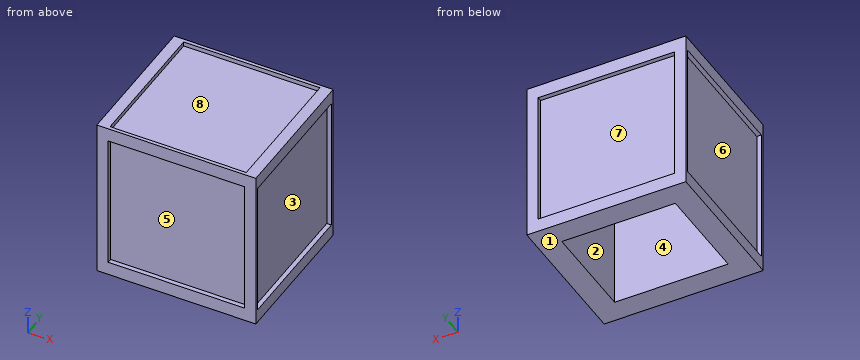
Autodesk Inventor part; units mm, degrees
ref_plane "YZ Plane" through (0, 0, 0) normal (1, 0, 0) x (0, 1, 0)
ref_plane "XZ Plane" through (0, 0, 0) normal (0, 1, 0) x (-1, 0, 0)
ref_plane "XY Plane" through (0, 0, 0) normal (0, 0, 1) x (1, 0, 0)
sketch "Sketch3" plane through (0, 0, 0) normal (0, 0, 1) x (1, 0, 0)
  line L0 (0, 0) -> (-50, 0)
  line L1 (-50, 0) -> (-50, 43)
  line L2 (-50, 43) -> (0, 43)
  line L3 (0, 43) -> (0, 0)
  line L4 (10, -10) -> (-60, -10)
  line L5 (-60, -10) -> (-60, 53)
  line L6 (-60, 53) -> (10, 53)
  line L7 (10, 53) -> (10, -10)
  dimension "d26" = 43
  dimension "d27" = 50
  dimension "d28" = 70
  dimension "d29" = 63
extrude "Extrusion3" add sketch "Sketch3" along normal blind 60
sketch "Sketch4" plane through (0, 0, 60) normal (0, 0, 1) x (1, 0, 0)
  line L0 (10, -10) -> (-60, -10)
  line L1 (-60, -10) -> (-60, 53)
  line L2 (-60, 53) -> (10, 53)
  line L3 (10, 53) -> (10, -10)
  point P0 (0, 0)
extrude "Extrusion4" add sketch "Sketch4" along normal blind 12
sketch "Sketch5" plane through (-60, 53, 0) normal (0, 1, 0) x (1, 0, 0)
  line L0 (0, 0) -> (70, 0)
  line L1 (70, 0) -> (70, -72)
  line L2 (0, 0) -> (70, 0)
  line L3 (70, 0) -> (70, -72)
  line L4 (70, -72) -> (0, -72)
  line L5 (0, -72) -> (0, 0)
  line L6 (65, -6) -> (5, -6)
  line L7 (5, -6) -> (5, -66)
  line L8 (5, -66) -> (65, -66)
  line L9 (65, -66) -> (65, -6)
  line L10 (60, -11) -> (10, -11)
  line L11 (10, -11) -> (10, -61)
  line L12 (10, -61) -> (60, -61)
  line L13 (60, -61) -> (60, -11)
  point P0 (60, 0)
  dimension "d34" = 60
  dimension "d35" = 60
  dimension "d36" = 50
  dimension "d37" = 50
extrude "Extrusion5" cut sketch "Sketch5" against normal blind 2 contours L9 L8 L7 L6 | L13 L12 L11 L10
sketch "Sketch6" plane through (10, -10, 0) normal (1, 0, 0) x (0, 0, -1)
  line L0 (-6, 1.5) -> (-66, 1.5)
  line L1 (-66, 1.5) -> (-66, 61.5)
  line L2 (-66, 61.5) -> (-6, 61.5)
  line L3 (-6, 61.5) -> (-6, 1.5)
  line L4 (-11, 6.5) -> (-61, 6.5)
  line L5 (-61, 6.5) -> (-61, 56.5)
  line L6 (-61, 56.5) -> (-11, 56.5)
  line L7 (-11, 56.5) -> (-11, 6.5)
  point P0 (0, 10)
  dimension "d40" = 60
  dimension "d41" = 60
  dimension "d42" = 50
  dimension "d43" = 50
extrude "Extrusion6" cut sketch "Sketch6" against normal blind 2 contours L0 L1 L2 L3 | L4 L5 L6 L7
sketch "Sketch7" plane through (-60, -10, 0) normal (0, -1, 0) x (1, 0, 0)
  line L0 (5, 6) -> (65, 6)
  line L1 (65, 6) -> (65, 66)
  line L2 (65, 66) -> (5, 66)
  line L3 (5, 66) -> (5, 6)
  line L4 (10, 11) -> (60, 11)
  line L5 (60, 11) -> (60, 61)
  line L6 (60, 61) -> (10, 61)
  line L7 (10, 61) -> (10, 11)
  point P0 (60, 0)
  dimension "d46" = 60
  dimension "d47" = 60
  dimension "d48" = 50
  dimension "d49" = 50
extrude "Extrusion7" cut sketch "Sketch7" against normal blind 2 contours L3 L2 L1 L0 | L7 L6 L5 L4
sketch "Sketch8" plane through (-60, -10, 0) normal (-1, 0, 0) x (0, 0, 1)
  line L0 (6, 1.5) -> (66, 1.5)
  line L1 (66, 1.5) -> (66, 61.5)
  line L2 (66, 61.5) -> (6, 61.5)
  line L3 (6, 61.5) -> (6, 1.5)
  line L4 (11, 6.5) -> (61, 6.5)
  line L5 (61, 6.5) -> (61, 56.5)
  line L6 (61, 56.5) -> (11, 56.5)
  line L7 (11, 56.5) -> (11, 6.5)
  point P0 (0, 10)
  dimension "d52" = 60
  dimension "d53" = 60
  dimension "d54" = 50
  dimension "d55" = 50
extrude "Extrusion8" cut sketch "Sketch8" against normal blind 2 contours L3 L2 L1 L0 | L7 L6 L5 L4
sketch "Sketch9" plane through (0, 0, 72) normal (0, 0, 1) x (1, 0, 0)
  line L0 (5, -8.5) -> (-55, -8.5)
  line L1 (-55, -8.5) -> (-55, 51.5)
  line L2 (-55, 51.5) -> (5, 51.5)
  line L3 (5, 51.5) -> (5, -8.5)
  line L4 (0, 46.5) -> (-50, 46.5)
  line L5 (-50, 46.5) -> (-50, -3.5)
  line L6 (-50, -3.5) -> (0, -3.5)
  line L7 (0, -3.5) -> (0, 46.5)
  point P0 (0, 0)
  dimension "d58" = 60
  dimension "d59" = 60
  dimension "d60" = 50
  dimension "d61" = 50
extrude "Extrusion9" cut sketch "Sketch9" against normal blind 2 contours L0 L1 L2 L3 | L7 L6 L5 L4
properties part number "End-Effector"
Work out the finished part from the listing and answer in its coordinate system (mm). Face numbers are marked on the shaded views. A direction names the side the tool comes from. Round coordinates to 2 decimals unless told otherwise and drop trailing zeros. Loops run counter-clockwise (first coordinate to the right, second up) from the corner with the lowest first, then second, coordinate; pieces in that order, holes last. Notation, with made-up numbers: (1, 52.5) - (58, 52.5) arc R13 cw to (58, 76.5) - close; hole circle Ø5 at (-20, -6.5). An arc over 180 degrees is marked (long way). One line per item, written item: value.
Q1. Straight lines are drawn through the part: probe 1 along Y at (x, z) = (-26, 22); probe 2 along X at (y, z) = (40, 53); probe 3 along X at (y, z) = (-2.5, 50). For each, find the intervals that lie inside material, in ascending order.
Check values:
probe 1: -8 to 0, 43 to 51
probe 2: -58 to -50, 0 to 8
probe 3: -58 to 8
Q2. For the marked faces 5, 6, 7 and 8, determine the directions among +Z, -Z, +X, -X, +Y, -Y from which every point of the face is accessible in a straight line to the end or side of a thin tool.
Check values:
face 5: -Y
face 6: -X
face 7: +Y
face 8: +Z
Q3. Find section B-B on x = 3.5. Give the vertices of the cut face in (y, z).
Check values:
outline: (-10, 0) - (53, 0) - (53, 6) - (51, 6) - (51, 66) - (53, 66) - (53, 72) - (51.5, 72) - (51.5, 70) - (-8.5, 70) - (-8.5, 72) - (-10, 72) - (-10, 66) - (-8, 66) - (-8, 6) - (-10, 6) - close
Q4. The mould has two halves that part along X. Classify the marked faces 1, 2, 3 and 4: +X half, -X half, draft (parallel to the pull), parting line (faces both ways), or undercut.
Check values:
face 1: draft
face 2: undercut
face 3: +X half
face 4: undercut
Q5. Find section A-A on z = 15.5. Give the vertices of the cut face in (x, y), and give its area (3 significant figures).
Check values:
outline: (-60, -10) - (-55, -10) - (-55, -8) - (5, -8) - (5, -10) - (10, -10) - (10, -8.5) - (8, -8.5) - (8, 51.5) - (10, 51.5) - (10, 53) - (5, 53) - (5, 51) - (-55, 51) - (-55, 53) - (-60, 53) - (-60, 51.5) - (-58, 51.5) - (-58, -8.5) - (-60, -8.5) - close; hole (-50, 0) - (0, 0) - (0, 43) - (-50, 43) - close
area: 1,780 mm2
Q6. Find section C-C on y = 5. Give the vertices of the cut face in (x, z).
Check values:
outline: (-60, 0) - (-50, 0) - (-50, 60) - (0, 60) - (0, 0) - (10, 0) - (10, 6) - (8, 6) - (8, 66) - (10, 66) - (10, 72) - (5, 72) - (5, 70) - (-55, 70) - (-55, 72) - (-60, 72) - (-60, 66) - (-58, 66) - (-58, 6) - (-60, 6) - close
Q7. Find section D-D on z = 63. Give the vertices of the cut face in (x, y), and give its area (3 significant figures).
Check values:
outline: (-60, -10) - (-55, -10) - (-55, -8) - (5, -8) - (5, -10) - (10, -10) - (10, -8.5) - (8, -8.5) - (8, 51.5) - (10, 51.5) - (10, 53) - (5, 53) - (5, 51) - (-55, 51) - (-55, 53) - (-60, 53) - (-60, 51.5) - (-58, 51.5) - (-58, -8.5) - (-60, -8.5) - close
area: 3,930 mm2
Q8. Each of these flat-tipped pins is pushed along its axis until it touches: pin 1 Ø18 at (x, z) = (-15.5, 41) entering from -Y; pin 2 Ø13 at (x, y) = (-33, 17.5) entering from -Z; pin 3 Ø1 at (x, y) = (-23, -2.5) entering from +Z. Where does it stop, or does it pass through?
Check values:
pin 1: y = -8
pin 2: z = 60
pin 3: z = 70
